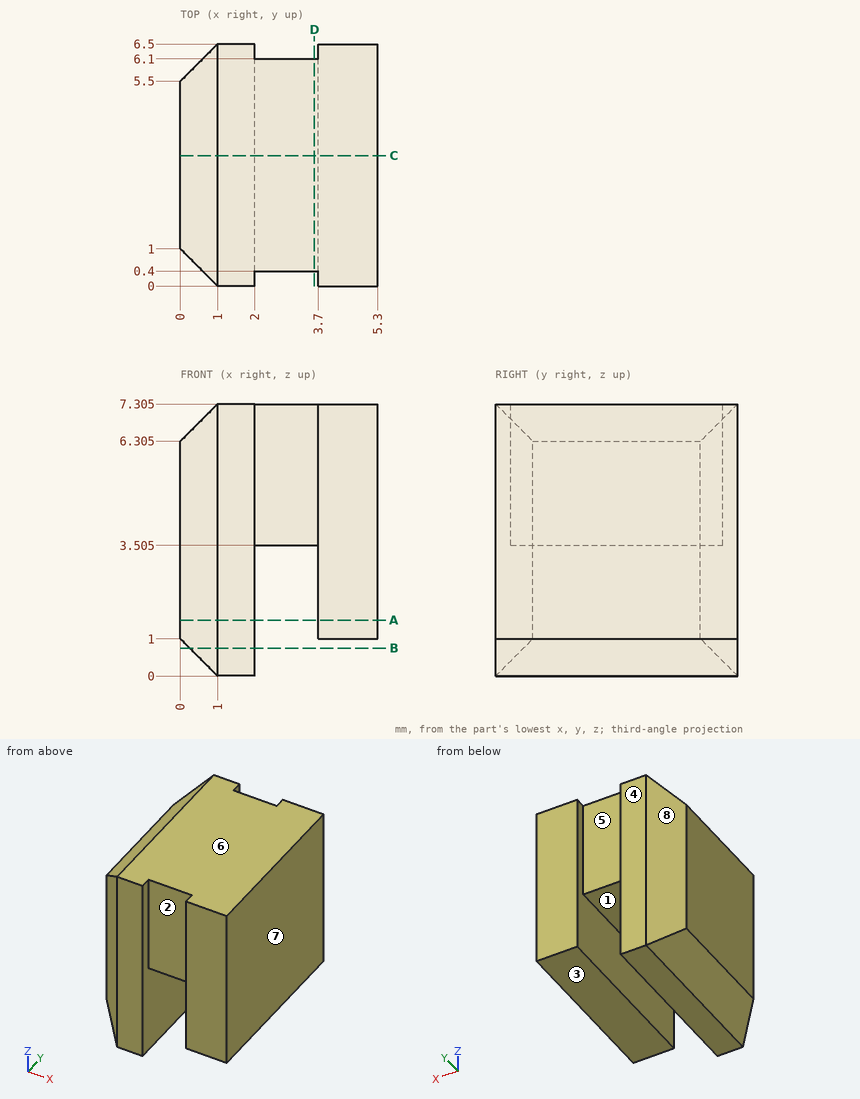
Design review of the part shown in the three views and the two pictorial views. Dimensions are in mm from the part's minimum x, y and z. A direction names the side the tool comes from. Coordinates: 2 decimals unless noted, no trailing zeros. Write each loop counter-clockwise with the first axis right and the second up, starting at its lowest first coordinate (ties: lowest second). Pieces come first, ordered by that corner, then holes.
(1) Add section A-A on z = 1.5. Give the boundary of the cut face in (x, y), then the cut area to 3 significant figures.
(2) Tool access review of the marked faces 1, 2, 3 and 4: name each direction out of +Z, -Z, +X, -X, +Y, -Y from which nothing blocks a thin tool from reaching the whole face with its end or side.
(3) For pin 1 Ø0.8 at (x, y) = (4, 4.5) entering from -Z, flat-tipped, find the tip position at first contact; note if it passes through.
(4) Wall thickness on probe 1 along X at (y, z) = (2.5, 3); probe 2 along Z at (x, y) = (4.7, 3.25) (3 decimals); probe 3 along Z at (x, y) = (2.75, 3.5) (3 decimals): over which ranges is each line inside the solid? List them lowest first.
(5) Add section B-B on z = 0.75. Give the boundary of the cut face in (x, y), then the cut area to 3 significant figures.
(6) Add section C-C on y = 3.5. Give the boundary of the cut face in (x, z) (3 decimals).
(7) The part is to be moulded in two halves that separate along X. For the marked faces 5, 6, 7 and 8, say which applies: +X half, -X half, draft (parallel to the pull), parting line (faces both ways), or undercut.
(8) Add section D-D on x = 3.6. Give the boundary of the cut face in (y, z) (3 decimals).
Answer sheet:
1. outline: (0, 1) - (1, 0) - (2, 0) - (2, 6.5) - (1, 6.5) - (0, 5.5) - close; (3.7, 0) - (5.3, 0) - (5.3, 6.5) - (3.7, 6.5) - close
1. area: 22.4 mm2
2. face 1: -Z, +Y, -Y
2. face 2: +Z, -Z, -Y
2. face 3: -Z, +X, +Y, -Y
2. face 4: +Z, -Z, +X, -X, +Y
3. pin 1: stops at z = 1
4. probe 1: x = 0 to 2, 3.7 to 5.3
4. probe 2: z = 1 to 7.305
4. probe 3: z = 3.505 to 7.305
5. outline: (0.25, 0.75) - (1, 0) - (2, 0) - (2, 6.5) - (1, 6.5) - (0.25, 5.75) - close
5. area: 10.8 mm2
6. outline: (0, 1) - (1, 0) - (2, 0) - (2, 3.505) - (3.7, 3.505) - (3.7, 1) - (5.3, 1) - (5.3, 7.305) - (1, 7.305) - (0, 6.305) - close
7. face 5: undercut
7. face 6: draft
7. face 7: +X half
7. face 8: -X half
8. outline: (0.4, 3.505) - (6.1, 3.505) - (6.1, 7.305) - (0.4, 7.305) - close
